from build123d import *

# Parameters (mm, degrees)
SKETCH1_W           = 28
SKETCH1_H           = 64.64
BOSS_EXTRUDE1_DEPTH = 3
SKETCH2_R           = 2.5
CUT_EXTRUDE1_DEPTH  = 71.507656322
SKETCH4_W           = 20.1
SKETCH4_H           = 40.64
CUT_EXTRUDE6_DEPTH  = 10
SKETCH5_W           = 28
SKETCH5_H           = 3
BOSS_EXTRUDE2_DEPTH = 16
SKETCH6_R           = 1
CUT_EXTRUDE7_DEPTH  = 10


with BuildPart() as part:
    # Sketch1 → Boss-Extrude1 (new body)
    with BuildSketch(Plane.XY):
        with Locations((14, 32.32)):
            Rectangle(SKETCH1_W, SKETCH1_H)
    extrude(amount=BOSS_EXTRUDE1_DEPTH)

    # Sketch2 → Cut-Extrude1 (cut, through all)
    with BuildSketch(Plane.XY.offset(3)):
        with Locations((9, 9.57)):
            Circle(SKETCH2_R)
        with Locations((19, 9.57)):
            Circle(SKETCH2_R)
        with Locations((9, 60.07)):
            Circle(SKETCH2_R)
        with Locations((19, 60.07)):
            Circle(SKETCH2_R)
    extrude(amount=-CUT_EXTRUDE1_DEPTH, mode=Mode.SUBTRACT)

    # Sketch4 → Cut-Extrude6 (cut)
    with BuildSketch(Plane.XY.offset(3)):
        with Locations((14, 34.82)):
            Rectangle(SKETCH4_W, SKETCH4_H)
    extrude(amount=-CUT_EXTRUDE6_DEPTH, mode=Mode.SUBTRACT)

    # Sketch5 → Boss-Extrude2 (add)
    with BuildSketch(Plane(origin=(0, 0, 0), x_dir=(-1, 0, 0), z_dir=(0, 0, -1))):
        with Locations((-14, 1.5)):
            Rectangle(SKETCH5_W, SKETCH5_H)
    extrude(amount=BOSS_EXTRUDE2_DEPTH)

    # Sketch6 → Cut-Extrude7 (cut)
    with BuildSketch(Plane(origin=(0, 3, 0), x_dir=(1, 0, 0), z_dir=(0, 1, 0))):
        with Locations(Location((5, 5.5, 0), (0, 0, 180))):
            Circle(SKETCH6_R)
        with Locations(Location((5, 13.5, 0), (0, 0, 180))):
            Circle(SKETCH6_R)
        with Locations(Location((23, 13.5, 0), (0, 0, 180))):
            Circle(SKETCH6_R)
        with Locations(Location((23, 5.5, 0), (0, 0, 180))):
            Circle(SKETCH6_R)
    extrude(amount=-CUT_EXTRUDE7_DEPTH, mode=Mode.SUBTRACT)


solid = part.part
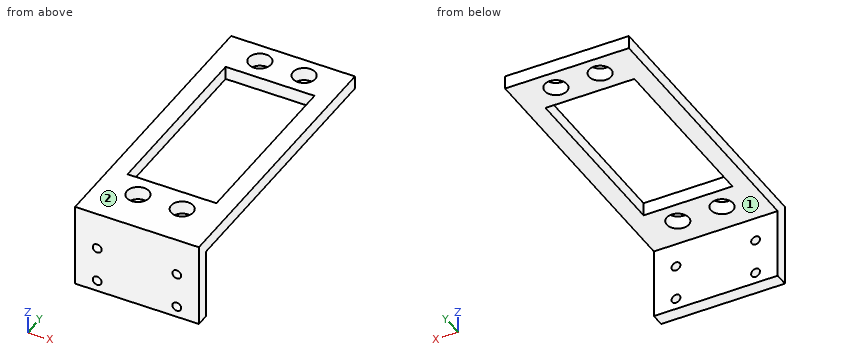
Part model, mm, in its own coordinate system. Face numbers are marked on the shaded views. A direction names the side the tool comes from. Give positions to 0.01 mm unless a question says otherwise; leave off trailing zeros. Write each loop counter-clockwise with the first axis right and the second up, starting at its lowest first coordinate (ties: lowest second). Pieces come first, ordered by that corner, then holes.
1) Cut at C-C on x = 5. Write the cut outline in (y, z).
Resolved:
outline: (0, -16) - (3, -16) - (3, -14.5) - (0, -14.5) - close; (0, -12.5) - (3, -12.5) - (3, -6.5) - (0, -6.5) - close; (0, -4.5) - (3, -4.5) - (3, 0) - (14.5, 0) - (14.5, 3) - (0, 3) - close; (55.14, 0) - (64.64, 0) - (64.64, 3) - (55.14, 3) - close
2) Which spindle directions (+Z, -Z, +X, -X, +Y, -Y) get a long thin tool onto all of the face, cutting with end or side? Do the marked faces 1 and 2. Say none if no direction does.
Resolved:
face 1: -Z, +X, -X, +Y
face 2: +Z, +X, -X, +Y, -Y
3) Cut at A-A on x = 15.25. Write the cut outline in (y, z).
Resolved:
outline: (0, -16) - (3, -16) - (3, 0) - (14.5, 0) - (14.5, 3) - (0, 3) - close; (55.14, 0) - (64.64, 0) - (64.64, 3) - (55.14, 3) - close
4) Cut at B-B on y = 26. Write the cut outline in (x, z).
Resolved:
outline: (0, 0) - (3.95, 0) - (3.95, 3) - (0, 3) - close; (24.05, 0) - (28, 0) - (28, 3) - (24.05, 3) - close
5) Pin check, flat tips, straight feed: pin 1 (3.5 mm diameter, centred on y = 25, z = 1, fed in from -X); pin 2 (8 mm diameter, centred on x = 10.5, z = -10.5, fed in from +Y); pin 3 (10 mm diameter, centred on y = 32, z = -8.5, fed in from -X); pin 4 (3 mm diameter, centred on x = 15, y = 7, fed in from -Z). Stop position of each tip, or through.
Resolved:
pin 1: stops at x = 0
pin 2: stops at y = 3
pin 3: passes through
pin 4: stops at z = 0
6) Cut at D-D on y = 9.57. Write the cut outline in (x, z).
Resolved:
outline: (0, 0) - (6.5, 0) - (6.5, 3) - (0, 3) - close; (11.5, 0) - (16.5, 0) - (16.5, 3) - (11.5, 3) - close; (21.5, 0) - (28, 0) - (28, 3) - (21.5, 3) - close
7) Probe L1, parallel to Y at x = 12, z = 1; L2, parallel to X at y = 26, z = 2.25; L3, parallel to X at y = 58, z = 2. List the from-to ranges inside material, lowest first.
Resolved:
L1: y = 0 to 14.5, 55.14 to 64.64
L2: x = 0 to 3.95, 24.05 to 28
L3: x = 0 to 7.6, 10.4 to 17.6, 20.4 to 28
